```python
from build123d import *

# Parameters (mm, degrees)
SKETCH_1_W             = 4.1
SKETCH_1_H             = 3
EXTRUDE_1_DEPTH        = 1.6
CHAMFER_1_SIZE         = 0.76
CHAMFER_1_SIZE2        = 0.8
EXTRUDE_2_DEPTH        = 0.15
PATTERN_LINEAR_1_COUNT = 2
PATTERN_LINEAR_1_PITCH = 1.3
MIRROR_1_COPY_1_DEPTH  = 0.15
MIRROR_1_COPY_2_DEPTH  = 0.15


with BuildPart() as part:
    # Эскиз1 → Бобышка-Вытянуть1 (new body)
    with BuildSketch(Plane(origin=(0, 0, 0), x_dir=(1, 0, 0), z_dir=(0, 1, 0))):
        Rectangle(SKETCH_1_W, SKETCH_1_H)
    extrude(amount=EXTRUDE_1_DEPTH)

    # Фаска1
    chamfer_1_edges = [part.edges().sort_by_distance(p)[0] for p in [
        (2.05, 0, 0),
        (-2.05, 0, 0),
    ]]
    chamfer_1_side = [part.faces().sort_by_distance(p)[0] for p in [
        (0, 0, 0),
    ]]
    chamfer(chamfer_1_edges, length=CHAMFER_1_SIZE, length2=CHAMFER_1_SIZE2, reference=chamfer_1_side[0])

    # Эскиз2 → Бобышка-Вытянуть2 (add, symmetric)
    with BuildSketch(Plane(origin=(0, 0, 0), x_dir=(0, 0, -1), z_dir=(1, 0, 0))):
        with BuildLine():
            Line((-2.2, 0.84), (-1.5, 0.84))
            Line((-1.5, 0.84), (-1.5, 0.54))
            Line((-1.5, 0.54), (-2.2, 0.54))
            ThreePointArc((-2.2, 0.54), (-2.907106781, 0.247106781), (-3.2, -0.46))
            Line((-3.2, -0.46), (-3.2, -13.16))
            Line((-3.2, -13.16), (-3.5, -13.16))
            Line((-3.5, -13.16), (-3.5, -0.46))
            ThreePointArc((-3.5, -0.46), (-3.119238816, 0.459238816), (-2.2, 0.84))
        make_face()
    extrude_2 = extrude(amount=EXTRUDE_2_DEPTH, both=True)

    # Линейный массив1: Бобышка-Вытянуть2 ×2
    with Locations(*[(-i * PATTERN_LINEAR_1_PITCH, 0, 0) for i in range(1, PATTERN_LINEAR_1_COUNT)]):
        add(extrude_2)

    # Зеркальное отражение1 copy 1 sketch → Зеркальное отражение1 copy 1 (add, symmetric)
    with BuildSketch(Plane(origin=(1.3, 0, 0), x_dir=(0, 0, -1), z_dir=(-1, 0, 0))):
        with BuildLine():
            Line((-2.2, -0.84), (-1.5, -0.84))
            Line((-1.5, -0.84), (-1.5, -0.54))
            Line((-1.5, -0.54), (-2.2, -0.54))
            ThreePointArc((-2.2, -0.54), (-2.907106781, -0.247106781), (-3.2, 0.46))
            Line((-3.2, 0.46), (-3.2, 13.16))
            Line((-3.2, 13.16), (-3.5, 13.16))
            Line((-3.5, 13.16), (-3.5, 0.46))
            ThreePointArc((-3.5, 0.46), (-3.119238816, -0.459238816), (-2.2, -0.84))
        make_face()
    extrude(amount=MIRROR_1_COPY_1_DEPTH, both=True)

    # Зеркальное отражение1 copy 2 sketch → Зеркальное отражение1 copy 2 (add, symmetric)
    with BuildSketch(Plane(origin=(0, 0, 0), x_dir=(0, 0, -1), z_dir=(-1, 0, 0))):
        with BuildLine():
            Line((-2.2, -0.84), (-1.5, -0.84))
            Line((-1.5, -0.84), (-1.5, -0.54))
            Line((-1.5, -0.54), (-2.2, -0.54))
            ThreePointArc((-2.2, -0.54), (-2.907106781, -0.247106781), (-3.2, 0.46))
            Line((-3.2, 0.46), (-3.2, 13.16))
            Line((-3.2, 13.16), (-3.5, 13.16))
            Line((-3.5, 13.16), (-3.5, 0.46))
            ThreePointArc((-3.5, 0.46), (-3.119238816, -0.459238816), (-2.2, -0.84))
        make_face()
    extrude(amount=MIRROR_1_COPY_2_DEPTH, both=True)


solid = part.part
```
For this review, take the finished solid that the model builds, in its own axes (mm). A direction names the side the tool comes from. Round coordinates to 2 decimals unless told otherwise and drop trailing zeros. Write each loop counter-clockwise with the first axis right and the second up, starting at its lowest first coordinate (ties: lowest second). Pieces come first, ordered by that corner, then holes. Notation, with made-up numbers: (23, -39) - (46, -39) arc R20 ccw to (46, -20) - close; hole circle Ø11 at (-32.75, 47.5). An arc over 180 degrees is marked (long way). Answer as CSV lines item,"result". Start each with the question number.
(1) Machinability: for faces 1 (the cylindrical face through (1.3, 0.45, 3.13)), 2 (the flat face through (0, 0, 0)), which of the approach directions +Z, -Z, +X, -X, +Y, -Y give a long, thin tool a straight path to every point of the face, cutting with its end or side? Answer none if there is none.
(2) Add section B-B, the plane y = -9. State the section outline as (x, z) points.
(3) For pin 1 (0.8 mm diameter, centred on x = 0, y = 1, fed in from +Z); pin 2 (0.6 mm diameter, centred on y = -5.5, z = 2.5, fed in from +X); pin 3 (1.6 mm diameter, centred on y = -6, z = 2.5, fed in from -X); pin 4 (1 mm diameter, centred on x = 1, z = -0.5, fed in from -Y), all flat-tipped, find the tip position at first contact; note any pin that passes through.
(4) Add section C-C, the plane z = -0.4. State the section outline as (x, y) points.
(5) For line 1 (Y direction, x = 1.25, z = -0.45); line 2 (Z direction, x = -1.2, y = -7.25); line 3 (Y direction, x = -1.8, z = -0.8), list the stretches that pass through material, from the lowest coordinate up.
(6) Add section A-A, the plane z = 1.7. State the section outline as (x, y) points.
(7) Add section D-D, the plane x = 0.6. State the section outline as (y, z) points.
From the geometry:
1,face 1,"+Z, +X, -X, +Y"
1,face 2,"-Z, +X, -X, -Y"
2,outline,"(-1.45, 3.2) - (-1.15, 3.2) - (-1.15, 3.5) - (-1.45, 3.5) - close; (-0.15, 3.2) - (0.15, 3.2) - (0.15, 3.5) - (-0.15, 3.5) - close; (1.15, 3.2) - (1.45, 3.2) - (1.45, 3.5) - (1.15, 3.5) - close"
3,pin 1,"stops at z = 2.95"
3,pin 2,"passes through"
3,pin 3,"stops at x = -1.45"
3,pin 4,"stops at y = 0"
4,outline,"(-2.05, 0.8) - (-1.29, 0) - (1.29, 0) - (2.05, 0.8) - (2.05, 1.6) - (-2.05, 1.6) - close"
5,line 1,"y = 0 to 1.6"
5,line 2,"z = 3.2 to 3.5"
5,line 3,"y = 0.54 to 1.6"
6,outline,"(-1.45, 0.54) - (-1.15, 0.54) - (-1.15, 0.84) - (-1.45, 0.84) - close; (-0.15, 0.54) - (0.15, 0.54) - (0.15, 0.84) - (-0.15, 0.84) - close; (1.15, 0.54) - (1.45, 0.54) - (1.45, 0.84) - (1.15, 0.84) - close"
7,outline,"(0, -1.5) - (1.6, -1.5) - (1.6, 1.5) - (0, 1.5) - close"
